Input: dimensioned drawing with shaded views. Units: mm. Origin: part minimum x, y, z. Coordinates: 2 decimals unless noted, no trailing zeros. Order: outer loops, then holes, each group sorted by start corner. A loop starts at its lowest first (then second) coordinate and runs counter-clockwise, first axis right, second up.
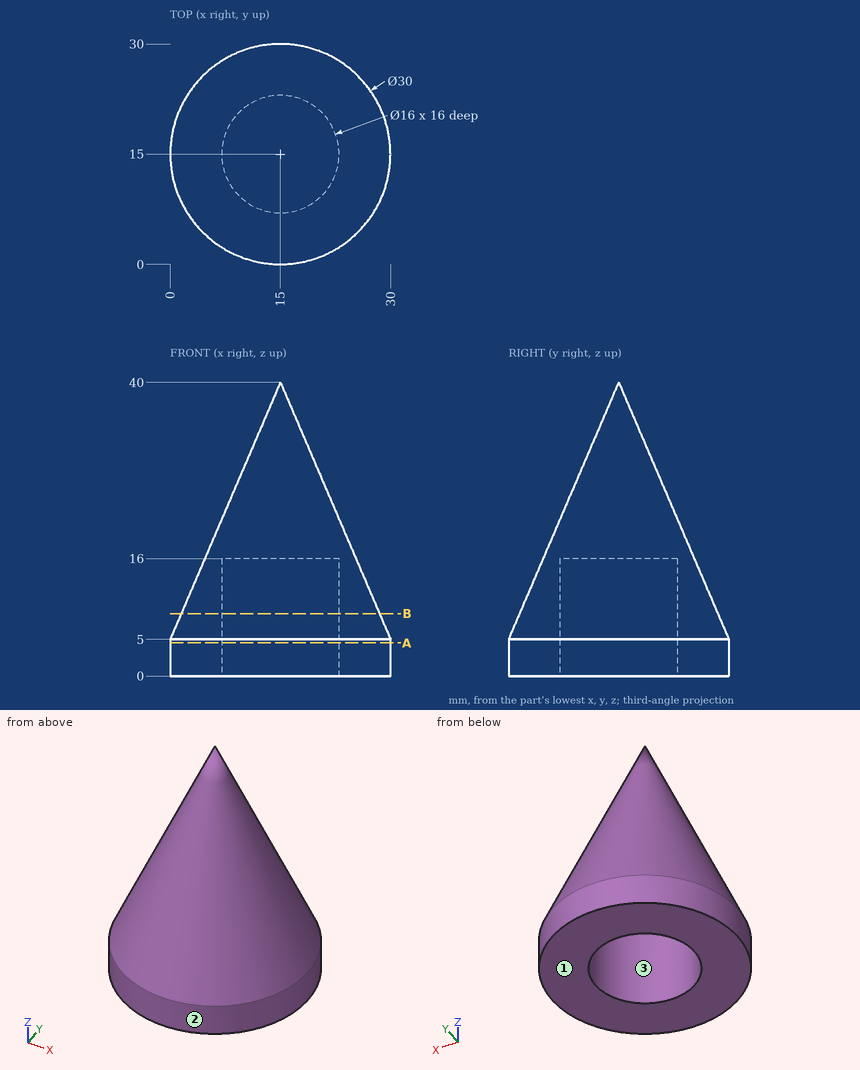
1. Ray query, line 1 (Y direction, x = 15, z = 4.25); line 2 (Y direction, x = 15, z = 5.75); line 3 (X direction, y = 13.75, z = 12). Return the intervals inside material, ascending.
Findings:
line 1: y = 0 to 7, 23 to 30
line 2: y = 0.32 to 7, 23 to 29.68
line 3: x = 3.07 to 7.1, 22.9 to 26.93
2. Section query B-B on z = 8.5. Return loops of the section in (x, y).
Findings:
outline: circle Ø27 at (15, 15); hole circle Ø16 at (15, 15)
3. Pin query (flat end, axial travel): P1, Ø10, axis at x = 12.5, z = 5, coming from the -Y side; P2, Ø5, axis at x = 23, y = 4, coming from the +Z side; P3, Ø5, axis at y = 12.5, z = 34.5, coming from the +X side; P4, Ø1, axis at x = 25.5, y = 16.5, coming from the +Z side. Return the tip coordinate at first contact, or that it passes through.
Findings:
P1: stops at y = 0
P2: stops at z = 14.1
P3: stops at x = 18.05
P4: stops at z = 16.42
4. Section query A-A on z = 4.5. Return loops of the section in (x, y), plus the area to 3 significant figures.
Findings:
outline: circle Ø30 at (15, 15); hole circle Ø16 at (15, 15)
area: 506 mm2
5. Draft query along Y for the marked faces 1, 2 and 3. Return one class per face: released by +Y, released by -Y, zero draft, split by the parting line, or undercut.
Findings:
face 1: zero draft
face 2: split by the parting line
face 3: undercut
